CAD build for the part. Positions are in the model's coordinates, mm. A direction names the side the tool comes from. Give positions to 0.01 mm unless a question says otherwise; leave off trailing zeros. Write each loop counter-clockwise with the first axis right and the second up, starting at its lowest first coordinate (ties: lowest second). Pieces come first, ordered by that corner, then holes. Notation, with made-up numbers: (62.25, 71.5) - (112.25, 71.5) arc R24 ccw to (112.25, 106.5) - close; hole circle Ø10 at (51, -32.75). An arc over 180 degrees is marked (long way). Answer as a JSON object with one key per item and string values.
from build123d import *

# Parameters (mm, degrees)
BOSS_EXTRUDE1_DEPTH = 3
SKETCH2_W           = 5
SKETCH2_H           = 3
CUT_EXTRUDE2_DEPTH  = 3


with BuildPart() as part:
    # Sketch1 → Boss-Extrude1 (new body)
    with BuildSketch(Plane.XY):
        Polygon((30, -11.75), (30, -4.25), (25, 0.95), (25, 13.75), (-12.692307692, 13.75), (-25, 0.95), (-30, -4.25), (-30, -11.75), (-34.5, -11.75), (-34.5, -14.75), (-30, -14.75), (-30, -16.75), (-20, -16.75), (-20, -4.25), (-17.115384615, -1.25), (17.115384615, -1.25), (20, -4.25), (20, -16.75), (30, -16.75), (30, -14.75), (34.5, -14.75), (34.5, -11.75), align=None)
    extrude(amount=BOSS_EXTRUDE1_DEPTH)

    # Sketch2 → Cut-Extrude2 (cut)
    with BuildSketch(Plane(origin=(0, 0, 3), x_dir=(-1, 0, 0), z_dir=(0, 0, -1))):
        with Locations((9.5, 4.217126269)):
            Rectangle(SKETCH2_W, SKETCH2_H)
        with Locations((9.5, 9.717126269)):
            Rectangle(SKETCH2_W, SKETCH2_H)
        with Locations((-20.5, 4.217126269)):
            Rectangle(SKETCH2_W, SKETCH2_H)
        with Locations((-20.5, 9.717126269)):
            Rectangle(SKETCH2_W, SKETCH2_H)
    extrude(amount=CUT_EXTRUDE2_DEPTH, mode=Mode.SUBTRACT)


solid = part.part
(1) Flat gauge pins, fed straight in: P1, Ø1.5, axis at x = -33, z = 1.5, coming from the -Y side; P2, Ø1.5, axis at x = -8.5, z = 1, coming from the -Y side; P3, Ø1.5, axis at y = -6.5, z = 2, coming from the +X side. Where does each tip first touch, or does it go through?
Answer key:
{"P1": "stops at y = -14.75", "P2": "stops at y = -1.25", "P3": "stops at x = 30"}
(2) Saw through at D-D, the plane x = 27.5. Give the cut face in (y, z).
Answer key:
{"outline": "(-16.75, 0) - (-1.65, 0) - (-1.65, 3) - (-16.75, 3) - close"}
(3) Probe L1, parallel to Y at x = -9, z = 1.35; L2, parallel to Y at x = 22, z = 1.45; L3, parallel to X at y = -7, z = 0.9. List the from-to ranges inside material, lowest first. Write a range as [from, to].
Answer key:
{"L1": "y = [-1.25, 2.72], [5.72, 8.22], [11.22, 13.75]", "L2": "y = [-16.75, 2.72], [5.72, 8.22], [11.22, 13.75]", "L3": "x = [-30, -20], [20, 30]"}
(4) Saw through at A-A, the plane y = -8. Give the cut face in (x, z).
Answer key:
{"outline": "(-30, 0) - (-20, 0) - (-20, 3) - (-30, 3) - close; (20, 0) - (30, 0) - (30, 3) - (20, 3) - close"}
(5) Saw through at C-C, the plane x = -14. Give the cut face in (y, z).
Answer key:
{"outline": "(-1.25, 0) - (12.39, 0) - (12.39, 3) - (-1.25, 3) - close"}
(6) Pull direction Y, two halves, no side cores. Call faces 6 (the face through (-9, 5.717, 2)), 7 (the face through (-32, -14.75, 1)), 8 (the face through (30, -16, 1)): pulls with the +Y half, pulls with the -Y half, needs draft (parallel to the pull), parting line crosses it, or undercut.
Answer key:
{"face 6": "undercut", "face 7": "pulls with the -Y half", "face 8": "needs draft"}
(7) Saw through at B-B, the plane z = 1.25. State how many separate pieces and enclosed holes the cut face has, and give its area (3 significant figures).
Answer key:
{"separate pieces": "1", "enclosed holes": "4", "area": "953 mm²"}
(8) 3-axis set-ups, long thin cutter, end or side, ignore diameter. For faces 1 (the face through (-30, -16, 1)), 2 (the face through (0, 2, 3)), 3 (the face through (0, -1.25, 1)), 4 (the face through (-30, -8, 1)), 5 (the face through (21, 8.217, 2)): which of +Z, -Z, +X, -X, +Y, -Y reach the whole face in a straight line?
Answer key:
{"face 1": "+Z, -Z, -X, -Y", "face 2": "+Z, +X, -X, +Y, -Y", "face 3": "+Z, -Z, -Y", "face 4": "+Z, -Z, -X, +Y", "face 5": "+Z, -Z"}
